Source: CAD feature listing. Evaluate the final solid. Frame: model axes, mm. Face numbers are marked on the shaded views. A direction names the side the tool comes from. Coordinates: 2 decimals unless noted, no trailing zeros. Order: outer loops, then holes, each group sorted by start corner. A loop starts at its lowest first (then second) coordinate and runs counter-clockwise, first axis right, second up. Notation, with made-up numbers: (50, 11) - (78, 11) arc R21 cw to (78, 22) - close; hole circle Ø1 at (-22.5, 84.5). An arc over 180 degrees is marked (long way). One line per question, with ' | ' between items.
Autodesk Inventor part; units mm, degrees
ref_plane "YZ Plane" through (0, 0, 0) normal (1, 0, 0) x (0, 1, 0)
ref_plane "XZ Plane" through (0, 0, 0) normal (0, 1, 0) x (-1, 0, 0)
ref_plane "XY Plane" through (0, 0, 0) normal (0, 0, 1) x (1, 0, 0)
sketch "Sketch1" plane through (0, 0, 0) normal (1, 0, 0) x (0, 1, 0)
  line L0 (0, 150) -> (0, -150) construction
  line L1 (-22.5, 150) -> (-22.5, -150)
  line L2 (22.5, -150) -> (22.5, 150)
  arc A0 (22.5, 150) -> (-22.5, 150) centre (0, 150) ccw
  arc A1 (-22.5, -150) -> (22.5, -150) centre (0, -150) ccw
  line L3 (27.5, 150) -> (27.5, -150)
  arc A2 (-27.5, -150) -> (27.5, -150) centre (0, -150) ccw
  line L4 (-27.5, -150) -> (-27.5, 150)
  arc A3 (27.5, 150) -> (-27.5, 150) centre (0, 150) ccw
  point P0 (0, 0)
  dimension "d0" = 150
  dimension "d1" = 45
  dimension "d2" = 5
extrude "Extrusion1" add sketch "Sketch1" along normal blind 100
properties part number "Conveyor Belt New" material "Rubber, Silicone"
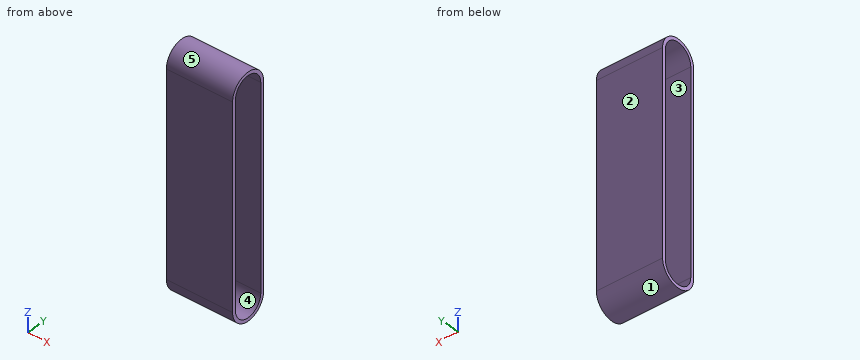
(1) Cut plane C-C (z = 134). Return the cut outline in (x, y).
Taken from the geometry:
outline: (0, -27.5) - (100, -27.5) - (100, -22.5) - (0, -22.5) - close; (0, 22.5) - (100, 22.5) - (100, 27.5) - (0, 27.5) - close
(2) Pin query (flat end, axial travel): P1, Ø1.5, axis at x = 56.5, y = 19, coming from the +Z side; P2, Ø1, axis at x = 19, y = -9.5, coming from the -Z side; P3, Ø2, axis at x = 43, y = 0.5, coming from the +Z side. Return the tip coordinate at first contact, or that it passes through.
Taken from the geometry:
P1: stops at z = 170.57 | P2: stops at z = -175.99 | P3: stops at z = 177.5
(3) Material intervals for L1, parallel to Y at x = 42, z = 47.5; L2, parallel to Z at x = 69.5, y = 1; L3, parallel to Z at x = 46, y = 15.5, sorted ascending. Write a range as from..to.
Taken from the geometry:
L1: y = -27.5..-22.5, 22.5..27.5 | L2: z = -177.48..-172.48, 172.48..177.48 | L3: z = -172.72..-166.31, 166.31..172.72
(4) Pull-direction query (Z, two-part tool) for the marked faces 1, 2 and 3; classes: pulls with the +Z half, pulls with the -Z half, needs draft (parallel to the pull), parting line crosses it, or undercut.
Taken from the geometry:
face 1: pulls with the -Z half | face 2: needs draft | face 3: undercut
(5) Cut plane A-A (x = 49.5). Return the cut outline in (y, z), and give its area (3 significant figures).
Taken from the geometry:
outline: (-27.5, -150) arc R27.5 ccw to (27.5, -150) - (27.5, 150) arc R27.5 ccw to (-27.5, 150) - close; hole (-22.5, -150) arc R22.5 ccw to (22.5, -150) - (22.5, 150) arc R22.5 ccw to (-22.5, 150) - close | area: 3,790 mm²
(6) Cut plane B-B (y = 0). Return the cut outline in (x, z), and give its area (3 significant figures).
Taken from the geometry:
outline: (0, -177.5) - (100, -177.5) - (100, -172.5) - (0, -172.5) - close; (0, 172.5) - (100, 172.5) - (100, 177.5) - (0, 177.5) - close | area: 1,000 mm²
(7) Set-up query: the marked faces 4 and 5. Return all of +Z, -Z, +X, -X, +Y, -Y with unobstructed straight access to the full face (end or side cutting, diameter ignored); none if empty.
Taken from the geometry:
face 4: +X, -X | face 5: +Z, +X, -X
